Part model, mm, in its own coordinate system. A direction names the side the tool comes from. Coordinates: 2 decimals unless noted, no trailing zeros. Loops run counter-clockwise (first coordinate to the right, second up) from the corner with the lowest first, then second, coordinate; pieces in that order, holes last. Notation, with made-up numbers: M -27.5,18.5 L 17.5,18.5 A21 ccw 17.5,25.5 Z; hole C 74,-19.5 d3. An arc over 180 degrees is marked long. Use CSV: the item, a comma, the result in double quotes. Start each with the question number.
from build123d import *

# Parameters (mm, degrees)
SKETCH_1_W              = 260
SKETCH_1_H              = 90
EXTRUDE_1_DEPTH         = 2
HOLE_WIZARD_4_2_4_2_1_D = 4.2
CUT_EXTRUDE_1_DEPTH     = 159.126531613
FILLET_1_R              = 4
FILLET_1_OF_MIRROR_2_R  = 4
CUT_EXTRUDE_2_DEPTH     = 159.126531613


with BuildPart() as part:
    # 草图1 → 凸台-拉伸1 (new body)
    with BuildSketch(Plane.XY):
        with Locations((0, 45)):
            Rectangle(SKETCH_1_W, SKETCH_1_H)
    extrude(amount=EXTRUDE_1_DEPTH)

    # Ø4.2 (4.2) 直径孔1 (through all)
    with Locations(Plane(origin=(-60, 5, 2), x_dir=(1, 0, 0), z_dir=(0, 0, 1))):
        with Locations((0, 0), (-25, 0)):
            hole_wizard_4_2_4_2_1 = Hole(HOLE_WIZARD_4_2_4_2_1_D / 2)

    # 镜向1: Ø4.2 (4.2) 直径孔1 across plane
    add(hole_wizard_4_2_4_2_1.mirror(Plane(origin=(0, 0, 0), x_dir=(0, 0, 1), z_dir=(1, 0, 0))), mode=Mode.SUBTRACT)

    # 草图5 → 切除-拉伸1 (cut, through all)
    with BuildSketch(Plane.XY.offset(2)):
        Polygon((-120, 80), (-100, 80), (-120, 60), align=None)
        Polygon((-120, 15), (-108.431457505, 15), (-43.431457505, 80), (-63.230447378, 80), (-120, 23.230447378), align=None)
        Polygon((-5.247691321, 50.30151519), (-40.549206511, 15), (-19.336003076, 15), (-5.247691321, 29.088311755), align=None)
        Polygon((-91.514718626, 80), (-120, 51.514718626), (-120, 31.715728753), (-71.715728753, 80), align=None)
        Polygon((-34.946176131, 80), (-99.946176131, 15), (-78.732972695, 15), (-13.732972695, 80), align=None)
        Polygon((-5.247691321, 80), (-70.247691321, 15), (-49.034487885, 15), (-5.247691321, 58.786796564), align=None)
    cut_extrude_1 = extrude(amount=-CUT_EXTRUDE_1_DEPTH, mode=Mode.SUBTRACT)

    # 圆角1
    fillet_1_edges = [part.edges().sort_by_distance(p)[0] for p in [
        (-5.247691321, 80, 1),
        (-5.247691321, 58.786796564, 1),
        (-49.034487885, 15, 1),
        (-70.247691321, 15, 1),
        (-91.514718626, 80, 1),
        (-71.715728753, 80, 1),
        (-120, 31.715728753, 1),
        (-120, 51.514718626, 1),
        (-120, 15, 1),
        (-120, 23.230447378, 1),
        (-63.230447378, 80, 1),
        (-43.431457505, 80, 1),
        (-108.431457505, 15, 1),
        (-5.247691321, 50.30151519, 1),
        (-5.247691321, 29.088311755, 1),
        (-19.336003076, 15, 1),
        (-40.549206511, 15, 1),
        (-34.946176131, 80, 1),
        (-13.732972695, 80, 1),
        (-78.732972695, 15, 1),
        (-99.946176131, 15, 1),
        (-120, 60, 1),
        (-120, 80, 1),
        (-100, 80, 1),
    ]]
    fillet(fillet_1_edges, radius=FILLET_1_R)

    # 镜向2: 切除-拉伸1 across plane
    add(cut_extrude_1.mirror(Plane(origin=(0, 0, 0), x_dir=(0, 0, 1), z_dir=(1, 0, 0))), mode=Mode.SUBTRACT)

    # 圆角1 of 镜向2
    fillet_1_of_mirror_2_edges = [part.edges().sort_by_distance(p)[0] for p in [
        (5.247691321, 80, 1),
        (5.247691321, 58.786796564, 1),
        (49.034487885, 15, 1),
        (70.247691321, 15, 1),
        (91.514718626, 80, 1),
        (71.715728753, 80, 1),
        (120, 31.715728753, 1),
        (120, 51.514718626, 1),
        (120, 15, 1),
        (120, 23.230447378, 1),
        (63.230447378, 80, 1),
        (43.431457505, 80, 1),
        (108.431457505, 15, 1),
        (5.247691321, 50.30151519, 1),
        (5.247691321, 29.088311755, 1),
        (19.336003076, 15, 1),
        (40.549206511, 15, 1),
        (34.946176131, 80, 1),
        (13.732972695, 80, 1),
        (78.732972695, 15, 1),
        (99.946176131, 15, 1),
        (120, 60, 1),
        (120, 80, 1),
        (100, 80, 1),
    ]]
    fillet(fillet_1_of_mirror_2_edges, radius=FILLET_1_OF_MIRROR_2_R)

    # 草图6 → 切除-拉伸2 (cut, through all)
    with BuildSketch(Plane.XY.offset(2)):
        with BuildLine():
            Line((-1.414213562, 24.436508139), (-7.436508139, 18.414213562))
            ThreePointArc((-7.436508139, 18.414213562), (-7.870053642, 16.234633135), (-6.022294577, 15))
            Line((-6.022294577, 15), (6.022294577, 15))
            ThreePointArc((6.022294577, 15), (7.870053642, 16.234633135), (7.436508139, 18.414213562))
            Line((7.436508139, 18.414213562), (1.414213562, 24.436508139))
            ThreePointArc((1.414213562, 24.436508139), (0, 25.022294577), (-1.414213562, 24.436508139))
        make_face()
    extrude(amount=-CUT_EXTRUDE_2_DEPTH, mode=Mode.SUBTRACT)


solid = part.part
1. Two-plate mould, pull along X, no slides. Class faces 1 (the face through (-96.1, 55.615, 1.014)), 2 (the face through (-2, 46, 2)): pulls with the +X half, pulls with the -X half, needs draft (parallel to the pull), parting line crosses it, or undercut.
2. Wall check: probe 1 along Y at (x, z) = (85, 0.7); probe 2 along Y at (x, z) = (48, 1.35); probe 3 along Y at (x, z) = (-29, 1.7). Give the ranges that are in metal, low to high.
3. Slice it at B-B, the plane x = -28. List the corners of the cut face in (y, z).
4. Slice it at C-C, the plane z = 1.4. State how many separate pieces and enclosed holes the cut face has, and give its area (3 significant figures).
5. Tool access for faces 3 (the face through (-22.75, 32.8, 1.01)), 4 (the face through (-2, 46, 0)): list every direction of +Z, -Z, +X, -X, +Y, -Y with a clear straight run to the whole face (end or side of a thin tool).
6. Slice it at A-A, the plane x = 41. List the corners of the cut face in (y, z), and give its area (3 significant figures).
Found:
1,face 1,"undercut"
1,face 2,"needs draft"
2,probe 1,"0 to 2.9, 7.1 to 15, 29.95 to 38.43, 58.23 to 66.72, 80 to 90"
2,probe 2,"0 to 16.04, 37.25 to 45.73, 66.95 to 90"
2,probe 3,"0 to 15, 26.55 to 35.03, 56.25 to 64.73, 80 to 90"
3,outline,"M 0,0 L 15,0 L 15,2 L 0,2 Z; M 27.55,0 L 36.03,0 L 36.03,2 L 27.55,2 Z; M 57.25,0 L 65.73,0 L 65.73,2 L 57.25,2 Z; M 80,0 L 90,0 L 90,2 L 80,2 Z"
4,separate pieces,"1"
4,enclosed holes,"17"
4,area,"13,200 mm^2"
5,face 3,"+Z, -Z"
5,face 4,"-Z, +X, -X, +Y, -Y"
6,outline,"M 0,0 L 23.03,0 L 23.03,2 L 0,2 Z; M 44.25,0 L 52.73,0 L 52.73,2 L 44.25,2 Z; M 73.95,0 L 90,0 L 90,2 L 73.95,2 Z"
6,area,"95.1 mm^2"
